For this review, take the finished solid that the model builds, in its own axes (mm). Face numbers are marked on the shaded views. Coordinates: 2 decimals unless noted, no trailing zeros. Order: outer loops, then holes, each group sorted by start corner. A loop starts at its lowest first (then second) coordinate and runs counter-clockwise, first axis right, second up. Notation, with made-up numbers: M 10.5,-3.5 L 51.5,-3.5 A14 cw 51.5,18.5 Z; hole C 62.5,19.5 d5. An arc over 180 degrees is marked long. Use CSV: the item, a comma, the result in double quotes.
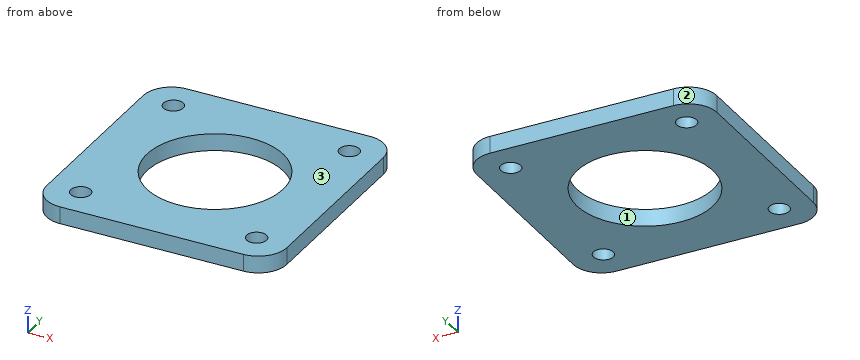
```python
from build123d import *

# Parameters (mm, degrees)
F0_R     = 1.75
F0_R_2   = 12
F1_DEPTH = 3


with BuildPart() as f1:
    # F0 (on Top) → F1 (new body)
    with BuildSketch(Plane.XY):
        with BuildLine():
            Line((31.65, 5.65), (-0.65, 5.65))
            ThreePointArc((-0.65, 5.65), (-4.185534, 4.185534), (-5.65, 0.65))
            Line((-5.65, 0.65), (-5.65, -31.65))
            ThreePointArc((-5.65, -31.65), (-4.185534, -35.185534), (-0.65, -36.65))
            Line((-0.65, -36.65), (31.65, -36.65))
            ThreePointArc((31.65, -36.65), (35.185534, -35.185534), (36.65, -31.65))
            Line((36.65, -31.65), (36.65, 0.65))
            ThreePointArc((36.65, 0.65), (35.185534, 4.185534), (31.65, 5.65))
        make_face()
        with Locations((0, -31)):
            Circle(F0_R, mode=Mode.SUBTRACT)
        with Locations((31, -31)):
            Circle(F0_R, mode=Mode.SUBTRACT)
        Circle(F0_R, mode=Mode.SUBTRACT)
        with Locations((15.5, -15.5)):
            Circle(F0_R_2, mode=Mode.SUBTRACT)
        with Locations((31, 0)):
            Circle(F0_R, mode=Mode.SUBTRACT)
    extrude(amount=F1_DEPTH)


solid = f1.part
```
Item 1: To check wall thickness, follow line 1 along Y through (x, z) = (31, 1.3); line 2 along X through (y, z) = (1, 0.95); line 3 along X through (y, z) = (-0.5, 1.9). State the ranges of each line that lie inside material, in increasing order. Write a range as [from, to].
Solutions:
line 1,"[-36.65, -32.75], [-29.25, -1.75], [1.75, 5.65]"
line 2,"[-5.64, -1.44], [1.44, 29.56], [32.44, 36.64]"
line 3,"[-5.65, -1.68], [1.68, 29.32], [32.68, 36.65]"
Item 2: Add section A-A on y = -15.5. State the section outline as (x, z) points.
Solutions:
outline,"M -5.65,0 L 3.5,0 L 3.5,3 L -5.65,3 Z; M 27.5,0 L 36.65,0 L 36.65,3 L 27.5,3 Z"
Item 3: Draft analysis for pull direction X (two halves, no side actions). For the marked faces 1, 2 and 3, state which applies: released by +X, released by -X, zero draft, split by the parting line, or undercut.
Solutions:
face 1,"undercut"
face 2,"released by -X"
face 3,"zero draft"
Item 4: Add section B-B on x = 31. State the section outline as (y, z) points, and give its area (3 significant figures).
Solutions:
outline,"M -36.65,0 L -32.75,0 L -32.75,3 L -36.65,3 Z; M -29.25,0 L -1.75,0 L -1.75,3 L -29.25,3 Z; M 1.75,0 L 5.65,0 L 5.65,3 L 1.75,3 Z"
area,"106 mm^2"
Item 5: Add section C-C on y = -31. State the section outline as (x, z) points, and give its area (3 significant figures).
Solutions:
outline,"M -5.65,0 L -1.75,0 L -1.75,3 L -5.65,3 Z; M 1.75,0 L 29.25,0 L 29.25,3 L 1.75,3 Z; M 32.75,0 L 36.65,0 L 36.65,3 L 32.75,3 Z"
area,"106 mm^2"
Item 6: Add section D-D on z = 1.15. State the section outline as (x, y) points, and give its area (3 significant figures).
Solutions:
outline,"M -5.65,-31.65 A5 ccw -0.65,-36.65 L 31.65,-36.65 A5 ccw 36.65,-31.65 L 36.65,0.65 A5 ccw 31.65,5.65 L -0.65,5.65 A5 ccw -5.65,0.65 Z; hole C 0,-31 d3.5; hole C 0,0 d3.5; hole C 15.5,-15.5 d24; hole C 31,-31 d3.5; hole C 31,0 d3.5"
area,"1,280 mm^2"
